Work out the finished part from the listing and answer in its coordinate system (mm). A direction names the side the tool comes from. Give positions to 0.01 mm unless a question says otherwise; leave off trailing zeros. Write each loop counter-clockwise with the first axis right and the second up, starting at its lowest first coordinate (ties: lowest second). Pieces come first, ordered by that corner, then holes.
1) Given pin 1 Ø3 at (x, z) = (8.5, 9) entering from +Y; pin 2 Ø5 at (x, z) = (-7, 2) entering from -Y, each flat-ended and moving along its own axis, determine where each tip first touches the part or whether it passes through.
2) Find section A-A (y = -5.5). Determine the outline of the cut face in (x, z).
3) A tool of negligible diameter and unlimited length cuts with its end or side. For faces 1 (the face through (7.39, -3.06, 4.93)), 2 (the face through (-0.1, 13.4, 2)), from which of +Z, -Z, +X, -X, +Y, -Y can it reach the whole face along a straight path? Write none if from no direction.
4) Find section C-C (y = 12). Determine the outline of the cut face in (x, z), plus the area to 3 significant figures.
5) Find section B-B (x = -4.5). Determine the outline of the cut face in (y, z).
6) Find section D-D (x = 11.5). Determine the outline of the cut face in (y, z).
7) Straight lines are drawn through the part: probe 1 along Y at (x, z) = (0, 2.25); probe 2 along X at (y, z) = (0, 6.75); probe 3 along Z at (x, y) = (5.5, 12). For each, find the intervals that lie inside material, in ascending order.
8) Determine the mould class of faces 3 (the face through (-10.17, 2.77, 3.85)), 4 (the face through (-14.985, 0.66, 0.986)), 5 (the face through (6, 6, 10)), 6 (the face through (6, -6, 0)) for opening direction Z: pulls with the +Z half, pulls with the -Z half, needs draft (parallel to the pull), parting line crosses it, or undercut.
```python
from build123d import *

# Parameters (mm, degrees)
F0_R     = 15
F0_R_2   = 8
F1_DEPTH = 2
F2_R     = 13
F2_R_2   = 8
F3_DEPTH = 8
F5_D     = 6
F5_DEPTH = 25
F5_TIP   = 1.8025818571


with BuildPart() as f1:
    # F0 (on Top) → F1 (new body)
    with BuildSketch(Plane.XY):
        Circle(F0_R)
        Circle(F0_R_2, mode=Mode.SUBTRACT)
    extrude(amount=F1_DEPTH)

    # F2 (on face) → F3 (join)
    with BuildSketch(Plane.XY.offset(2)):
        Circle(F2_R)
        Circle(F2_R_2, mode=Mode.SUBTRACT)
    extrude(amount=F3_DEPTH)

    # F5 (one way)
    with BuildSketch(Plane.YZ):
        with Locations((0, 5)):
            Circle(F5_D / 2)
    extrude(amount=-F5_DEPTH, mode=Mode.SUBTRACT)
    with Locations(Plane.YZ):
        with Locations((0, 5)):
            with Locations((0, 0, -(F5_DEPTH + F5_TIP / 2))):  # 118° drill point
                Cone(0, F5_D / 2, F5_TIP, mode=Mode.SUBTRACT)


solid = f1.part
```
Results:
1. pin 1: stops at y = 10.95
1. pin 2: stops at y = -14.31
2. outline: (-13.96, 0) - (-5.81, 0) - (-5.81, 10) - (-11.78, 10) - (-11.78, 2) - (-13.96, 2) - close; (5.81, 0) - (13.96, 0) - (13.96, 2) - (11.78, 2) - (11.78, 10) - (5.81, 10) - close
3. face 1: +Z, -Z
3. face 2: +Z
4. outline: (-9, 0) - (9, 0) - (9, 2) - (5, 2) - (5, 10) - (-5, 10) - (-5, 2) - (-9, 2) - close
4. area: 116 mm2
5. outline: (-14.31, 0) - (-6.61, 0) - (-6.61, 10) - (-12.2, 10) - (-12.2, 2) - (-14.31, 2) - close; (6.61, 0) - (14.31, 0) - (14.31, 2) - (12.2, 2) - (12.2, 10) - (6.61, 10) - close
6. outline: (-9.63, 0) - (9.63, 0) - (9.63, 2) - (6.06, 2) - (6.06, 10) - (-6.06, 10) - (-6.06, 2) - (-9.63, 2) - close
7. probe 1: y = -13 to -8, 8 to 13
7. probe 2: x = 8 to 13
7. probe 3: z = 0 to 2
8. face 3: undercut
8. face 4: needs draft
8. face 5: pulls with the +Z half
8. face 6: pulls with the -Z half
